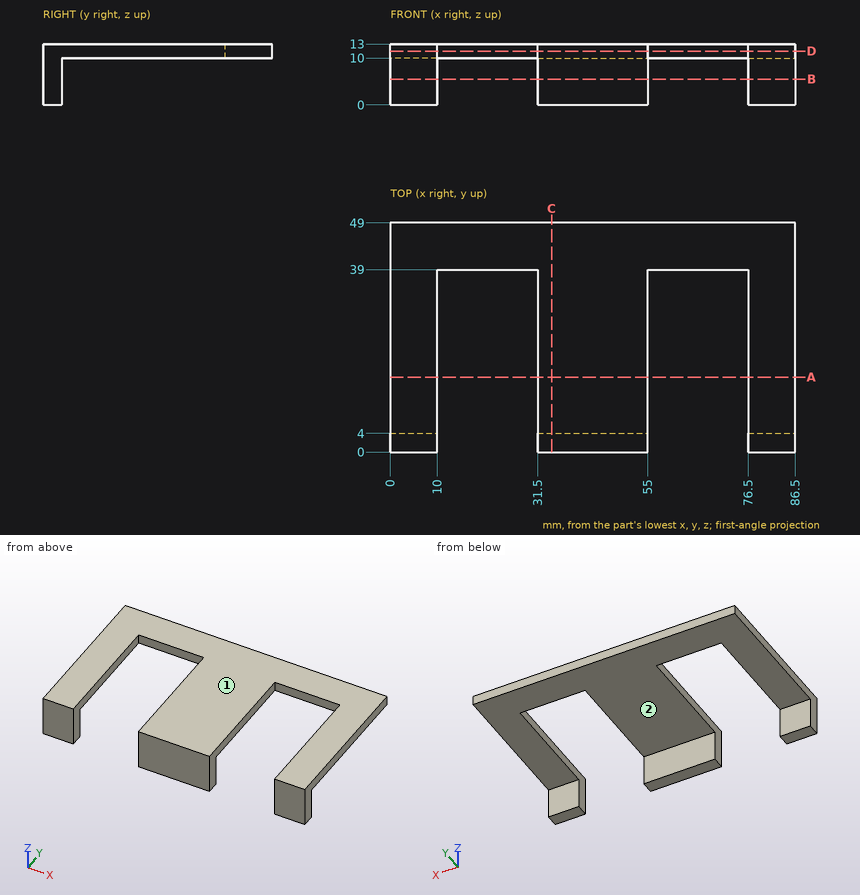
Check sheet for the drawn part. Datum: minimum x, y, z corner. Units: mm. A direction names the side the tool comes from. Give positions to 0.01 mm unless a question says otherwise; leave off trailing zeros. Loops run counter-clockwise (first coordinate to the right, second up) from the corner with the lowest first, then second, coordinate; pieces in that order, holes last. Notation, with made-up numbers: M -10.5,38 L 29.5,38 A20 cw 29.5,75 Z; hole C 39,41.25 d2. An arc over 180 degrees is marked long. Return JSON: item names as keys, results as strings.
1) Section check B-B, the plane z = 5.5. Enter the section's corners in (x, y), and give its area (3 significant figures).
Findings:
{"outline": "M 0,0 L 10,0 L 10,4 L 0,4 Z; M 31.5,0 L 55,0 L 55,4 L 31.5,4 Z; M 76.5,0 L 86.5,0 L 86.5,4 L 76.5,4 Z", "area": "174 mm2"}
2) Section check C-C, the plane x = 34.5. Enter the section's corners in (y, z).
Findings:
{"outline": "M 0,0 L 4,0 L 4,10 L 49,10 L 49,13 L 0,13 Z"}
3) Tool access check on the marked faces 1 and 2. Record the directions out of +Z, -Z, +X, -X, +Y, -Y that give a thin tool (end or side, any length) a straight path to the whole face; none if there is none.
Findings:
{"face 1": "+Z, +X, -X, +Y, -Y", "face 2": "-Z, +X, -X, +Y"}
4) Section check D-D, the plane z = 11.5. Enter the section's corners in (x, y).
Findings:
{"outline": "M 0,0 L 10,0 L 10,39 L 31.5,39 L 31.5,0 L 55,0 L 55,39 L 76.5,39 L 76.5,0 L 86.5,0 L 86.5,49 L 0,49 Z"}
5) Material ranges on L1, parallel to X at y = 22, z = 11; L2, parallel to Z at x = 46, y = 16; L3, parallel to Y at x = 50, z = 8.75, recorded low to high. Write a range as [from, to].
Findings:
{"L1": "x = [0, 10], [31.5, 55], [76.5, 86.5]", "L2": "z = [10, 13]", "L3": "y = [0, 4]"}
6) Gauge pin test, flat ends, axial feed: P1, Ø1.5, axis at x = 36, y = 15.5, coming from the -Z side; P2, Ø3, axis at x = 82.5, z = 3.5, coming from the +Y side; P3, Ø1.5, axis at x = 68, z = 11, coming from the -Y side. Record the tip position at first contact, or that the pin passes through.
Findings:
{"P1": "stops at z = 10", "P2": "stops at y = 4", "P3": "stops at y = 39"}
7) Section check A-A, the plane y = 16. Enter the section's corners in (x, z).
Findings:
{"outline": "M 0,10 L 10,10 L 10,13 L 0,13 Z; M 31.5,10 L 55,10 L 55,13 L 31.5,13 Z; M 76.5,10 L 86.5,10 L 86.5,13 L 76.5,13 Z"}
